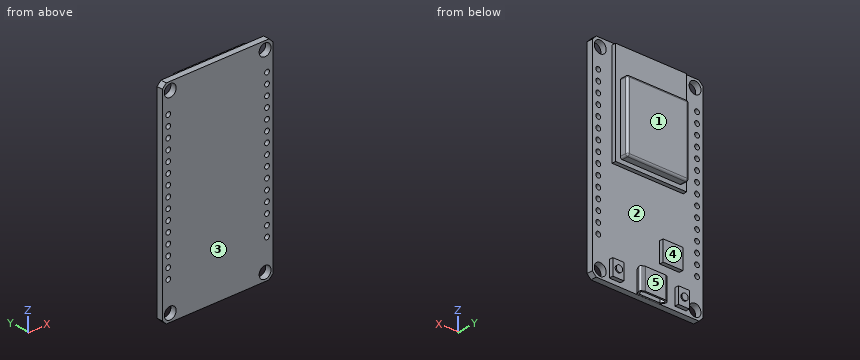
from build123d import *

# Parameters (mm, degrees)
ESBO_O2_R                = 1.5
RESSALTO_EXTRUS_O1_DEPTH = 1.5
ESBO_O3_W                = 18
ESBO_O3_H                = 25.5
RESSALTO_EXTRUS_O2_DEPTH = 1
ESBO_O4_W                = 15.6
ESBO_O4_H                = 17.5
RESSALTO_EXTRUS_O3_DEPTH = 2
ESBO_O5_W                = 5
ESBO_O5_H                = 5
ESBO_O5_W_2              = 2.8
ESBO_O5_H_2              = 4
RESSALTO_EXTRUS_O4_DEPTH = 1
ESBO_O6_R                = 0.8
RESSALTO_EXTRUS_O5_DEPTH = 0.3
RESSALTO_EXTRUS_O6_DEPTH = 5.4
ESBO_O8_W                = 7.643027542
ESBO_O8_H                = 2.610064774
CORTE_EXTRUS_O1_DEPTH    = 0.01
CORTE_EXTRUS_O2_DEPTH    = 5
ESBO_O11_R               = 0.6
CORTE_EXTRUS_O3_DEPTH    = 5
FILETE1_R                = 0.5


with BuildPart() as part:
    # Esboço2 → Ressalto-extrusão1 (new body)
    with BuildSketch(Plane(origin=(0, 0, 0), x_dir=(1, 0, 0), z_dir=(0, 1, 0))):
        Polygon((-14, -25), (-13, -26), (13, -26), (14, -25), (14, 25), (13, 26), (-13, 26), (-14, 25), align=None)
        with Locations(Location((-12, 24, 0), (0, 0, 270))):
            Circle(ESBO_O2_R, mode=Mode.SUBTRACT)
        with Locations(Location((12, 24, 0), (0, 0, 270))):
            Circle(ESBO_O2_R, mode=Mode.SUBTRACT)
        with Locations(Location((-12, -24, 0), (0, 0, 270))):
            Circle(ESBO_O2_R, mode=Mode.SUBTRACT)
        with Locations(Location((12, -24, 0), (0, 0, 270))):
            Circle(ESBO_O2_R, mode=Mode.SUBTRACT)
    extrude(amount=RESSALTO_EXTRUS_O1_DEPTH)

    # Esboço3 → Ressalto-extrusão2 (add)
    with BuildSketch(Plane(origin=(0, 1.5, 0), x_dir=(1, 0, 0), z_dir=(0, 1, 0))):
        with Locations((0, -12.75)):
            Rectangle(ESBO_O3_W, ESBO_O3_H)
    extrude(amount=RESSALTO_EXTRUS_O2_DEPTH)

    # Esboço4 → Ressalto-extrusão3 (add)
    with BuildSketch(Plane(origin=(0, 2.5, 0), x_dir=(1, 0, 0), z_dir=(0, 1, 0))):
        with Locations((0, -9.75)):
            Rectangle(ESBO_O4_W, ESBO_O4_H)
    extrude(amount=RESSALTO_EXTRUS_O3_DEPTH)

    # Esboço5 → Ressalto-extrusão4 (add)
    with BuildSketch(Plane(origin=(0, 1.5, 0), x_dir=(1, 0, 0), z_dir=(0, 1, 0))):
        with Locations((-5.523603775, 14.812859986)):
            Rectangle(ESBO_O5_W, ESBO_O5_H)
        with Locations((-8.3, 23)):
            Rectangle(ESBO_O5_W_2, ESBO_O5_H_2)
        with Locations((8.3, 23)):
            Rectangle(ESBO_O5_W_2, ESBO_O5_H_2)
    extrude(amount=RESSALTO_EXTRUS_O4_DEPTH)

    # Esboço6 → Ressalto-extrusão5 (add)
    with BuildSketch(Plane(origin=(0, 2.5, 0), x_dir=(1, 0, 0), z_dir=(0, 1, 0))):
        with Locations(Location((-8.3, 23, 0), (0, 0, 270))):
            Circle(ESBO_O6_R)
        with Locations(Location((8.3, 23, 0), (0, 0, 270))):
            Circle(ESBO_O6_R)
    extrude(amount=RESSALTO_EXTRUS_O5_DEPTH)

    # Esboço7 → Ressalto-extrusão6 (add)
    with BuildSketch(Plane(origin=(0, 0, -26), x_dir=(-1, 0, 0), z_dir=(0, 0, -1))):
        with BuildLine():
            Line((3.017267899, 1.5), (-2.682732101, 1.5))
            Line((-2.682732101, 1.5), (-3.241687067, 2.54804056))
            ThreePointArc((-3.241687067, 2.54804056), (-3.277055187, 2.934679492), (-3.025084898, 3.230063212))
            Line((-3.025084898, 3.230063212), (-2.594089093, 3.446728534))
            ThreePointArc((-2.594089093, 3.446728534), (-2.484917853, 3.48649988), (-2.369514792, 3.5))
            Line((-2.369514792, 3.5), (2.704050589, 3.5))
            ThreePointArc((2.704050589, 3.5), (2.81945365, 3.48649988), (2.928624891, 3.446728534))
            Line((2.928624891, 3.446728534), (3.359620695, 3.230063212))
            ThreePointArc((3.359620695, 3.230063212), (3.611590984, 2.934679492), (3.576222864, 2.54804056))
            Line((3.576222864, 2.54804056), (3.017267899, 1.5))
        make_face()
    extrude(amount=-RESSALTO_EXTRUS_O6_DEPTH)

    # Esboço8 → Corte-extrusão1 (cut)
    with BuildSketch(Plane(origin=(0, 0, -26), x_dir=(-1, 0, 0), z_dir=(0, 0, -1))):
        with Locations((-0.089109416, 2.805032387)):
            Rectangle(ESBO_O8_W, ESBO_O8_H)
    extrude(amount=-CORTE_EXTRUS_O1_DEPTH, mode=Mode.SUBTRACT)

    # Esboço10 → Corte-extrusão2 (cut)
    with BuildSketch(Plane(origin=(0, 0, -25.99), x_dir=(-1, 0, 0), z_dir=(0, 0, -1))):
        with BuildLine():
            Line((2.704050589, 3.1), (-2.369514792, 3.1))
            ThreePointArc((-2.369514792, 3.1), (-2.392595404, 3.097299976), (-2.414429652, 3.089345707))
            Line((-2.414429652, 3.089345707), (-2.845425456, 2.872680384))
            ThreePointArc((-2.845425456, 2.872680384), (-2.895819514, 2.813603641), (-2.88874589, 2.736275854))
            Line((-2.88874589, 2.736275854), (-2.442732101, 1.9))
            Line((-2.442732101, 1.9), (2.777267899, 1.9))
            Line((2.777267899, 1.9), (3.223281688, 2.736275854))
            ThreePointArc((3.223281688, 2.736275854), (3.230355312, 2.813603641), (3.179961254, 2.872680384))
            Line((3.179961254, 2.872680384), (2.748965449, 3.089345707))
            ThreePointArc((2.748965449, 3.089345707), (2.727131201, 3.097299976), (2.704050589, 3.1))
        make_face()
    extrude(amount=-CORTE_EXTRUS_O2_DEPTH, mode=Mode.SUBTRACT)

    # Esboço11 → Corte-extrusão3 (cut)
    with BuildSketch(Plane(origin=(0, 1.5, 0), x_dir=(1, 0, 0), z_dir=(0, 1, 0))):
        with Locations(Location((-12.5, 16.56, 0), (0, 0, 270))):
            Circle(ESBO_O11_R)
        with Locations(Location((-12.5, 14.02, 0), (0, 0, 270))):
            Circle(ESBO_O11_R)
        with Locations(Location((-12.5, 11.48, 0), (0, 0, 270))):
            Circle(ESBO_O11_R)
        with Locations(Location((-12.5, 8.94, 0), (0, 0, 270))):
            Circle(ESBO_O11_R)
        with Locations(Location((-12.5, 6.4, 0), (0, 0, 270))):
            Circle(ESBO_O11_R)
        with Locations(Location((-12.5, 3.86, 0), (0, 0, 270))):
            Circle(ESBO_O11_R)
        with Locations(Location((-12.5, 1.32, 0), (0, 0, 270))):
            Circle(ESBO_O11_R)
        with Locations(Location((-12.5, -1.22, 0), (0, 0, 270))):
            Circle(ESBO_O11_R)
        with Locations(Location((-12.5, -3.76, 0), (0, 0, 270))):
            Circle(ESBO_O11_R)
        with Locations(Location((-12.5, -6.3, 0), (0, 0, 270))):
            Circle(ESBO_O11_R)
        with Locations(Location((-12.5, -8.84, 0), (0, 0, 270))):
            Circle(ESBO_O11_R)
        with Locations(Location((-12.5, -11.38, 0), (0, 0, 270))):
            Circle(ESBO_O11_R)
        with Locations(Location((-12.5, -13.92, 0), (0, 0, 270))):
            Circle(ESBO_O11_R)
        with Locations(Location((-12.5, -16.46, 0), (0, 0, 270))):
            Circle(ESBO_O11_R)
        with Locations(Location((-12.5, -19, 0), (0, 0, 270))):
            Circle(ESBO_O11_R)
        with Locations(Location((12.5, -19, 0), (0, 0, 270))):
            Circle(ESBO_O11_R)
        with Locations(Location((12.5, -16.46, 0), (0, 0, 270))):
            Circle(ESBO_O11_R)
        with Locations(Location((12.5, -13.92, 0), (0, 0, 270))):
            Circle(ESBO_O11_R)
        with Locations(Location((12.5, -11.38, 0), (0, 0, 270))):
            Circle(ESBO_O11_R)
        with Locations(Location((12.5, -8.84, 0), (0, 0, 270))):
            Circle(ESBO_O11_R)
        with Locations(Location((12.5, -6.3, 0), (0, 0, 270))):
            Circle(ESBO_O11_R)
        with Locations(Location((12.5, -3.76, 0), (0, 0, 270))):
            Circle(ESBO_O11_R)
        with Locations(Location((12.5, -1.22, 0), (0, 0, 270))):
            Circle(ESBO_O11_R)
        with Locations(Location((12.5, 1.32, 0), (0, 0, 270))):
            Circle(ESBO_O11_R)
        with Locations(Location((12.5, 3.86, 0), (0, 0, 270))):
            Circle(ESBO_O11_R)
        with Locations(Location((12.5, 6.4, 0), (0, 0, 270))):
            Circle(ESBO_O11_R)
        with Locations(Location((12.5, 8.94, 0), (0, 0, 270))):
            Circle(ESBO_O11_R)
        with Locations(Location((12.5, 11.48, 0), (0, 0, 270))):
            Circle(ESBO_O11_R)
        with Locations(Location((12.5, 14.02, 0), (0, 0, 270))):
            Circle(ESBO_O11_R)
        with Locations(Location((12.5, 16.56, 0), (0, 0, 270))):
            Circle(ESBO_O11_R)
    extrude(amount=-CORTE_EXTRUS_O3_DEPTH, mode=Mode.SUBTRACT)

    # Filete1
    filete1_edges = [part.edges().sort_by_distance(p)[0] for p in [
        (7.8, 3.5, 18.5),
        (7.8, 3.5, 1),
        (-7.8, 3.5, 1),
        (-7.8, 3.5, 18.5),
        (7.8, 4.5, 9.75),
        (0, 4.5, 1),
        (-7.8, 4.5, 9.75),
        (0, 4.5, 18.5),
    ]]
    fillet(filete1_edges, radius=FILETE1_R)


solid = part.part
For this review, take the finished solid that the model builds, in its own axes (mm). Face numbers are marked on the shaded views. A direction names the side the tool comes from. Round coordinates to 2 decimals unless told otherwise and drop trailing zeros. Write each loop counter-clockwise with the first axis right and the second up, starting at its lowest first coordinate (ties: lowest second). Pieces come first, ordered by that corner, then holes. Notation, with made-up numbers: (-30.75, 89) - (-23.75, 89) arc R20 ccw to (-23.75, 119) - close; hole circle Ø8 at (8, 88). An arc over 180 degrees is marked (long way). Use a Markdown table: item, result.
Q1. We need section C-C (z = 11.38). Give the boundary of the cut face in (x, y), plus the area to 3 significant figures.
Derived:
| item | result |
|---|---|
| outline | (-14, 0) - (-13.1, 0) - (-13.1, 1.5) - (-14, 1.5) - close; (-11.9, 0) - (11.9, 0) - (11.9, 1.5) - (9, 1.5) - (9, 2.5) - (7.8, 2.5) - (7.8, 4) arc R0.5 ccw to (7.3, 4.5) - (-7.3, 4.5) arc R0.5 ccw to (-7.8, 4) - (-7.8, 2.5) - (-9, 2.5) - (-9, 1.5) - (-11.9, 1.5) - close; (13.1, 0) - (14, 0) - (14, 1.5) - (13.1, 1.5) - close |
| area | 87.5 mm2 |
Q2. We need section D-D (y = 0.75). State how many separate pieces and enclosed holes the cut face has, plus the area to 3 significant figures.
Derived:
| item | result |
|---|---|
| separate pieces | 1 |
| enclosed holes | 34 |
| area | 1,390 mm2 |
Q3. We need section A-A (z = -8.94). Give the boundary of the cut face in (x, y), plus the area to 3 significant figures.
Derived:
| item | result |
|---|---|
| outline | (-14, 0) - (-13.1, 0) - (-13.1, 1.5) - (-14, 1.5) - close; (-11.9, 0) - (11.9, 0) - (11.9, 1.5) - (-11.9, 1.5) - close; (13.1, 0) - (14, 0) - (14, 1.5) - (13.1, 1.5) - close |
| area | 38.4 mm2 |
Q4. Machinability: for the marked faces 3, 4 and 5, which of the approach directions +Z, -Z, +X, -X, +Y, -Y give a long, thin tool a straight path to every point of the face, cutting with its end or side? Answer none if there is none.
Derived:
| item | result |
|---|---|
| face 3 | +Z, -Z, +X, -X, -Y |
| face 4 | +X, -X, +Y |
| face 5 | -Z, +X, -X, +Y |
Q5. Wall thickness on line 1 along X through (y, z) = (0.95, -8.94); line 2 along X through (y, z) = (0.45, 8.5); line 3 along X through (y, z) = (1.9, 11): over which ranges is each line inside the solid? List them lowest first.
Derived:
| item | result |
|---|---|
| line 1 | x = -14 to -13.1, -11.9 to 11.9, 13.1 to 14 |
| line 2 | x = -14 to -12.99, -12.01 to 12.01, 12.99 to 14 |
| line 3 | x = -9 to 9 |
Q6. The part is to be moulded in two halves that separate along Z. For the marked faces 1 and 2, say which applies: pulls with the +Z half, pulls with the -Z half, needs draft (parallel to the pull), parting line crosses it, or undercut.
Derived:
| item | result |
|---|---|
| face 1 | needs draft |
| face 2 | undercut |
Q7. Clearance check with flat-ended pins moving along their axes: pin 1 (0.8 mm diameter, centred on y = 2, z = 14, fed in from -X); pin 2 (1 mm diameter, centred on x = 3, z = -2.5, fed in from +Y); pin 3 (0.8 mm diameter, centred on x = 8.5, z = -23.5, fed in from +Y). State where each tip first meets the part, or that it passes through.
Derived:
| item | result |
|---|---|
| pin 1 | stops at x = -9 |
| pin 2 | stops at y = 1.5 |
| pin 3 | stops at y = 2.8 |
